```python
from build123d import *

# Parameters (mm, degrees)
SKIZZE1_W                      = 57
SKIZZE1_H                      = 59
GRUNDK_RPER_DEPTH              = 2
SKIZZE2_R                      = 9.25
SKIZZE2_R_2                    = 1.6
BOHRUNGEN_KUGELROLLER_DEPTH    = 66.553413336
SKIZZE3_W                      = 10
SKIZZE3_H                      = 30
AUFSATZ_GETRIEBEHALTER_DEPTH   = 2
SKIZZE4_R                      = 1.6
BOHRUNGEN_GETRIEBEHALTER_DEPTH = 66.644877942
SKIZZE5_R                      = 1.6
BOHRUNG_HALTERUNG_DEPTH        = 66.553413336


with BuildPart() as part:
    # Skizze1 → Grundkörper (new body)
    with BuildSketch(Plane.XY):
        with Locations((0, 29.5)):
            Rectangle(SKIZZE1_W, SKIZZE1_H)
    extrude(amount=GRUNDK_RPER_DEPTH)

    # Skizze2 → Bohrungen_Kugelroller (cut, through all)
    with BuildSketch(Plane(origin=(0, 0, 0), x_dir=(-1, 0, 0), z_dir=(0, 0, -1))):
        with Locations((0, 47.75)):
            Circle(SKIZZE2_R)
        with Locations((-17.5, 47.75)):
            Circle(SKIZZE2_R_2)
        with Locations(Location((17.5, 47.75, 0), (0, 0, 180))):
            Circle(SKIZZE2_R_2)
    extrude(amount=-BOHRUNGEN_KUGELROLLER_DEPTH, mode=Mode.SUBTRACT)

    # Skizze3 → Aufsatz_Getriebehalter (add)
    with BuildSketch(Plane(origin=(0, 0, 0), x_dir=(-1, 0, 0), z_dir=(0, 0, -1))):
        with Locations((-23.5, 15)):
            Rectangle(SKIZZE3_W, SKIZZE3_H)
        with Locations((23.5, 15)):
            Rectangle(SKIZZE3_W, SKIZZE3_H)
    extrude(amount=AUFSATZ_GETRIEBEHALTER_DEPTH)

    # Skizze4 → Bohrungen_Getriebehalter (cut, through all)
    with BuildSketch(Plane(origin=(0, 0, -2), x_dir=(-1, 0, 0), z_dir=(0, 0, -1))):
        with Locations((-23.5, 26)):
            Circle(SKIZZE4_R)
        with Locations(Location((23.5, 26, 0), (0, 0, 180))):
            Circle(SKIZZE4_R)
        with Locations((23.5, 4)):
            Circle(SKIZZE4_R)
        with Locations(Location((-23.5, 4, 0), (0, 0, 180))):
            Circle(SKIZZE4_R)
    extrude(amount=-BOHRUNGEN_GETRIEBEHALTER_DEPTH, mode=Mode.SUBTRACT)

    # Skizze5 → Bohrung_Halterung (cut, through all)
    with BuildSketch(Plane(origin=(0, 0, 0), x_dir=(-1, 0, 0), z_dir=(0, 0, -1))):
        with Locations((0, 3)):
            Circle(SKIZZE5_R)
    extrude(amount=-BOHRUNG_HALTERUNG_DEPTH, mode=Mode.SUBTRACT)


solid = part.part
```
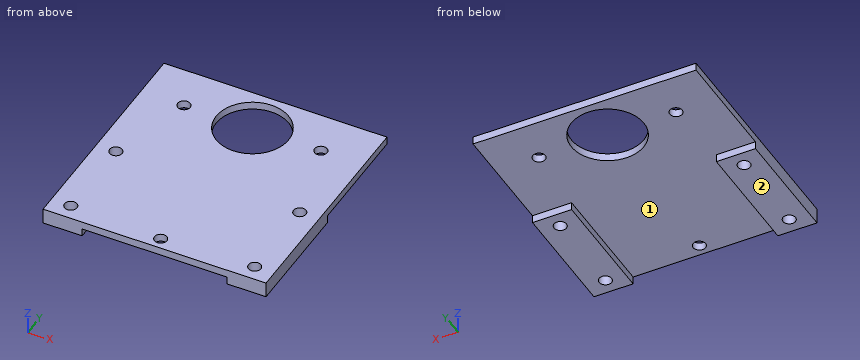
Work out the finished part from the listing and answer in its coordinate system (mm). Face numbers are marked on the shaded views. Give positions to 0.01 mm unless a question says otherwise; leave off trailing zeros. Loops run counter-clockwise (first coordinate to the right, second up) from the corner with the lowest first, then second, coordinate; pieces in that order, holes last. Notation, with made-up numbers: (30.5, -20.5) -> (46.5, -20.5) arc R28 ccw to (46.5, 6.5) -> close; hole circle Ø9 at (44, 22). An arc over 180 degrees is marked (long way). Put each result on its own line as item: value. Start each with the question number.
Item 1: The part is cut by section D-D (x = -3). Give the vertices of the cut face in (y, z).
Item 2: The part is cut by section C-C (y = 10.5). Give the vertices of the cut face in (x, z), then the cut area to 3 significant figures.
Item 3: The mould has two halves that part along X. Classify the marked faces 1 and 2: released by +X, released by -X, zero draft, split by the parting line, or undercut.
Item 4: The part is cut by section B-B (x = -23.5). Give the vertices of the cut face in (y, z).
Item 5: Each of these flat-tipped pins is pushed along its axis until it touches: P1, Ø0.6, axis at x = 24.5, z = -1, coming from the +Y side; P2, Ø4, axis at x = -17.5, y = 47.75, coming from the -Z side; P3, Ø1.9, axis at x = 23.5, y = 4, coming from the +Z side. Where does it stop, or does it pass through?
Item 6: The part is cut by section A-A (z = -1.3). Give the vertices of the cut face in (x, y).
Item 7: Find the intervals of material crossed by L1, parallel to Y at x = 23.5, z = -0.4; L2, parallel to Y at x = -23.5, z = 0.6; L3, parallel to X at y = 10.5, z = -0.1, in increasing order. Write a range as [from, to].
Answers below:
1. outline: (0, 0) -> (39, 0) -> (39, 2) -> (0, 2) -> close; (56.5, 0) -> (59, 0) -> (59, 2) -> (56.5, 2) -> close
2. outline: (-28.5, -2) -> (-18.5, -2) -> (-18.5, 0) -> (18.5, 0) -> (18.5, -2) -> (28.5, -2) -> (28.5, 2) -> (-28.5, 2) -> close
2. area: 154 mm2
3. face 1: undercut
3. face 2: zero draft
4. outline: (0, -2) -> (2.4, -2) -> (2.4, 2) -> (0, 2) -> close; (5.6, -2) -> (24.4, -2) -> (24.4, 2) -> (5.6, 2) -> close; (27.6, -2) -> (30, -2) -> (30, 0) -> (59, 0) -> (59, 2) -> (27.6, 2) -> close
5. P1: y = 30
5. P2: z = 0
5. P3: through
6. outline: (-28.5, 0) -> (-18.5, 0) -> (-18.5, 30) -> (-28.5, 30) -> close; (18.5, 0) -> (28.5, 0) -> (28.5, 30) -> (18.5, 30) -> close; hole circle Ø3.2 at (-23.5, 4); hole circle Ø3.2 at (-23.5, 26); hole circle Ø3.2 at (23.5, 4); hole circle Ø3.2 at (23.5, 26)
7. L1: [0, 2.4], [5.6, 24.4], [27.6, 30]
7. L2: [0, 2.4], [5.6, 24.4], [27.6, 59]
7. L3: [-28.5, -18.5], [18.5, 28.5]
